from build123d import *

# Parameters (mm, degrees)
F0_W     = 5.21
F0_H     = 2
F1_DEPTH = 2.28


with BuildPart() as f1:
    # F0 (on Top) → F1 (new body)
    with BuildSketch(Plane.XY):
        Polygon((12.053386, -12.54), (5.908386, -12.54), (5.908386, -22.02), (14.518386, -22.02), (14.518386, -12.54), align=None)
        with Locations((10.213386, -19.34)):
            Rectangle(F0_W, F0_H, mode=Mode.SUBTRACT)
        Polygon((-2.141614, -22.02), (-2.141614, -12.54), (-8.186614, -12.54), (-10.751614, -12.54), (-10.751614, -22.02), align=None)
        with Locations((-6.446614, -19.34)):
            Rectangle(F0_W, F0_H, mode=Mode.SUBTRACT)
        Polygon((-8.186614, -12.54), (-8.186614, -10.24), (-10.751614, -12.54), align=None)
        Polygon((-2.141614, -2.45), (-6.031614, -2.45), (-8.186614, -2.45), (-8.186614, -10.24), (-8.186614, -12.54), (-2.141614, -12.54), align=None)
        Polygon((-6.031614, -2.45), (-6.031614, -0.15), (-8.186614, -2.45), align=None)
        Polygon((6.608386, 0), (-2.701614, 0), (-2.701614, 8.22), (-6.031614, 8.22), (-6.031614, -0.15), (-6.031614, -2.45), (-2.141614, -2.45), (-2.141614, -1.51), (5.908386, -1.51), (5.908386, -2.45), (9.938386, -2.45), (9.938386, -0.15), (9.938386, 8.22), (6.608386, 8.22), align=None)
        Polygon((12.053386, -2.45), (9.938386, -2.45), (5.908386, -2.45), (5.908386, -12.54), (12.053386, -12.54), (12.053386, -10.24), align=None)
        Polygon((12.053386, -2.45), (9.938386, -0.15), (9.938386, -2.45), align=None)
        Polygon((14.518386, -12.54), (12.053386, -10.24), (12.053386, -12.54), align=None)
    extrude(amount=F1_DEPTH)


solid = f1.part
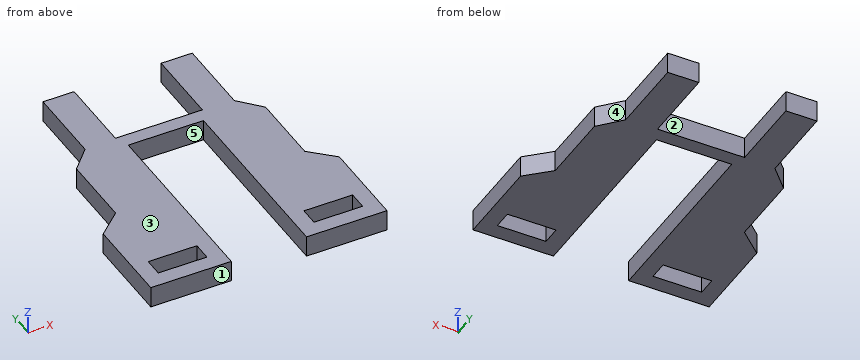
The model under review builds one solid part; all positions refer to its coordinate system, in mm. Face numbers are marked on the shaded views. A direction names the side the tool comes from. Give positions to 0.01 mm unless a question says otherwise; leave off trailing zeros. Order: outer loops, then holes, each group sorted by start corner. A loop starts at its lowest first (then second) coordinate and runs counter-clockwise, first axis right, second up. Notation, with made-up numbers: M 24.25,-0.75 L 50.25,-0.75 A16 ccw 50.25,22.25 Z; hole C 51.25,60.5 d1. An arc over 180 degrees is marked long. Use one line per item in the form item = value. Start each with the question number.
Item 1: The part is to be moulded in two halves that separate along X. For the marked faces 3, 4 and 5, say which applies: pulls with the +X half, pulls with the -X half, needs draft (parallel to the pull), parting line crosses it, or undercut.
Item 2: We need section A-A on y = -6. Give the boundary of the cut face in (x, z), plus the area to 3 significant figures.
Item 3: We need section B-B on x = 9.5. Give the boundary of the cut face in (y, z), plus the area to 3 significant figures.
Item 4: To check wall thickness, follow line 1 along X through (y, z) = (-16.5, 1.45); line 2 along X through (y, z) = (-2.5, 2.1); line 3 along Y through (x, z) = (9.5, 0.3). State the ranges of each line that lie inside material, in increasing order. Write a range as from..to.
Item 5: We need section D-D on x = 5.25. Give the boundary of the cut face in (y, z), plus the area to 3 significant figures.
Item 6: We need section C-C on z = 1.3. Give the boundary of the cut face in (x, y), plus the area to 3 significant figures.
Item 7: For the marked faces 1 and 2, list the 3-axis set-ups (+Z, -Z, +X, -X, +Y, -Y) from which the entire face can be reached by the end or side of a thin tool; tool diameter is ignored.
Item 8: Insertion check: pin 1 Ø0.7 at (y, z) = (-6, 1) entering from -X; pin 2 Ø1.1 at (x, z) = (2, 1) entering from -Y; pin 3 Ø1 at (y, z) = (-3, 1.5) entering from +X; pin 4 Ø12 at (x, y) = (0, -14.5) entering from -Z. Each pin has a flat end and moves straight along its axis. Give the tip position at first contact, or say it passes through.
Completed:
q1.face_3 = needs draft
q1.face_4 = pulls with the +X half
q1.face_5 = undercut
q2.outline = M -8.19,0 L -2.14,0 L -2.14,2.28 L -8.19,2.28 Z; M 5.91,0 L 12.05,0 L 12.05,2.28 L 5.91,2.28 Z
q2.area = 27.8 mm²
q3.outline = M -22.02,0 L -20.34,0 L -20.34,2.28 L -22.02,2.28 Z; M -18.34,0 L 8.22,0 L 8.22,2.28 L -18.34,2.28 Z
q3.area = 64.4 mm²
q4.line_1 = -10.75..-2.14, 5.91..14.52
q4.line_2 = -8.19..-2.14, 5.91..12.05
q4.line_3 = -22.02..-20.34, -18.34..8.22
q5.outline = M -1.51,0 L 0,0 L 0,2.28 L -1.51,2.28 Z
q5.area = 3.44 mm²
q6.outline = M -10.75,-22.02 L -2.14,-22.02 L -2.14,-1.51 L 5.91,-1.51 L 5.91,-22.02 L 14.52,-22.02 L 14.52,-12.54 L 12.05,-10.24 L 12.05,-2.45 L 9.94,-0.15 L 9.94,8.22 L 6.61,8.22 L 6.61,0 L -2.7,0 L -2.7,8.22 L -6.03,8.22 L -6.03,-0.15 L -8.19,-2.45 L -8.19,-10.24 L -10.75,-12.54 Z; hole M -9.05,-20.34 L -3.84,-20.34 L -3.84,-18.34 L -9.05,-18.34 Z; hole M 7.61,-20.34 L 12.82,-20.34 L 12.82,-18.34 L 7.61,-18.34 Z
q6.area = 362 mm²
q7.face_1 = +Z, -Z, +X, -X, -Y
q7.face_2 = +Z, -Z, +Y
q8.pin_1 = -8.19
q8.pin_2 = -1.51
q8.pin_3 = 12.05
q8.pin_4 = 0
